The model under review builds one solid part; all positions refer to its coordinate system, in mm. Round coordinates to 2 decimals unless told otherwise and drop trailing zeros. Order: outer loops, then holes, each group sorted by start corner. A loop starts at its lowest first (then second) coordinate and runs counter-clockwise, first axis right, second up. Notation, with made-up numbers: M 82.5,13.25 L 124.5,13.25 A23 ccw 124.5,28.25 Z; hole C 31.5,62 d10. An arc over 180 degrees is marked long. One line per item, written item: value. Start each with the question number.
from build123d import *

# Parameters (mm, degrees)
SKETCH1_R           = 16.9
BOSS_EXTRUDE1_DEPTH = 42.5
CHAMFER1_SIZE       = 2
CHAMFER2_SIZE       = 2


with BuildPart() as part:
    # Sketch1 → Boss-Extrude1 (new, symmetric)
    with BuildSketch(Plane.XY):
        Circle(SKETCH1_R)
    extrude(amount=BOSS_EXTRUDE1_DEPTH, both=True)

    # Chamfer1
    chamfer1_edges = [part.edges().sort_by_distance(p)[0] for p in [
        (-16.9, 0, 42.5),
    ]]
    chamfer(chamfer1_edges, length=CHAMFER1_SIZE)

    # Chamfer2
    chamfer2_edges = [part.edges().sort_by_distance(p)[0] for p in [
        (-16.9, 0, -42.5),
    ]]
    chamfer(chamfer2_edges, length=CHAMFER2_SIZE)


solid = part.part
Item 1: Wall thickness on L1, parallel to Y at x = 15.5, z = 26.5; L2, parallel to X at y = -1.5, z = -30; L3, parallel to Y at x = -7, z = 10: over which ranges is each line inside the solid? List them lowest first.
Item 2: Clearance check with flat-ended pins moving along their axes: P1, Ø6, axis at y = -11, z = -16, coming from the -X side; P2, Ø2, axis at x = 12.5, z = -12, coming from the +Y side; P3, Ø1, axis at x = -9, z = -2, coming from the -Y side. State where each tip first meets the part, or that it passes through.
Item 3: Consider section A-A, the plane z = -35. Give the boundary of the cut face in (x, y).
Computed:
1. L1: y = -6.73 to 6.73
1. L2: x = -16.83 to 16.83
1. L3: y = -15.38 to 15.38
2. P1: stops at x = -14.89
2. P2: stops at y = 12.38
2. P3: stops at y = -14.61
3. outline: C 0,0 d33.8
